Source: CAD feature listing. Evaluate the final solid. Frame: model axes, mm. Give positions to 0.01 mm unless a question says otherwise; leave off trailing zeros. Order: outer loops, then holes, each group sorted by start corner. A loop starts at its lowest first (then second) coordinate and runs counter-clockwise, first axis right, second up.
from build123d import *

# Parameters (mm, degrees)
ESQUISSE1_W             = 40
ESQUISSE1_H             = 17
BOSS_EXTRU_1_DEPTH      = 1
ENL_V_MAT_EXTRU_1_REACH = 45.474
ESQUISSE2_R             = 2.5
BOSS_EXTRU_2_DEPTH      = 8


with BuildPart() as part:
    # Esquisse1 → Boss.-Extru.1 (new body)
    with BuildSketch(Plane.XY):
        with Locations((20, 8.5)):
            Rectangle(ESQUISSE1_W, ESQUISSE1_H)
    extrude(amount=BOSS_EXTRU_1_DEPTH)

    # Esquisse2 → Enlèv. mat.-Extru.1 (cut, up to next)
    with BuildSketch(Plane.XY.offset(1), mode=Mode.PRIVATE) as enl_v_mat_extru_1_sk1:
        with Locations((6.5, 10.5)):
            Circle(ESQUISSE2_R)
    enl_v_mat_extru_1_tool1 = extrude(enl_v_mat_extru_1_sk1.sketch, amount=-ENL_V_MAT_EXTRU_1_REACH, mode=Mode.PRIVATE) & part.part
    # Esquisse2 → Enlèv. mat.-Extru.1 (cut, up to next)
    with BuildSketch(Plane.XY.offset(1), mode=Mode.PRIVATE) as enl_v_mat_extru_1_sk2:
        with Locations((33.5, 10.5)):
            Circle(ESQUISSE2_R)
    enl_v_mat_extru_1_tool2 = extrude(enl_v_mat_extru_1_sk2.sketch, amount=-ENL_V_MAT_EXTRU_1_REACH, mode=Mode.PRIVATE) & part.part
    add(enl_v_mat_extru_1_tool1.solids().sort_by_distance((6.5, 10.5, 1))[0], mode=Mode.SUBTRACT)
    add(enl_v_mat_extru_1_tool2.solids().sort_by_distance((33.5, 10.5, 1))[0], mode=Mode.SUBTRACT)

    # Esquisse3 → Boss.-Extru.2 (add)
    with BuildSketch(Plane.ZY.offset(-8)):
        with BuildLine():
            Line((0, 0), (0, -2))
            ThreePointArc((0, -2), (3.414213562, -3.414213562), (2, 0))
            Line((2, 0), (2, -1))
            ThreePointArc((2, -1), (2.707106781, -2.707106781), (1, -2))
            Line((1, -2), (1, 0))
            Line((1, 0), (0, 0))
        make_face()
    boss_extru_2 = extrude(amount=BOSS_EXTRU_2_DEPTH)

    # Symétrie1: Boss.-Extru.2 across plane
    add(boss_extru_2.mirror(Plane.ZY.offset(-20)))


solid = part.part
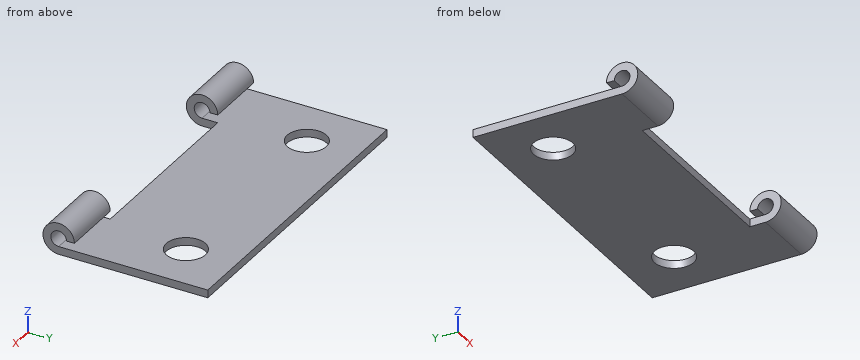
1) Ray query, L1, parallel to Z at x = 35.25, y = -2; L2, parallel to X at y = -1.25, z = 3.35; L3, parallel to Z at x = 37.5, y = 0.75. Return the intervals inside material, ascending.
Checks:
L1: z = 0 to 1, 3 to 4
L2: x = 0 to 8, 32 to 40
L3: z = 0 to 1
2) Section query C-C on z = 3.4. Output: boundary loops of the cut face in (x, y), and give its area (3 significant figures).
Checks:
outline: (0, -3.43) - (8, -3.43) - (8, -0.57) - (0, -0.57) - close; (32, -3.43) - (40, -3.43) - (40, -0.57) - (32, -0.57) - close
area: 45.7 mm2
3) Section query A-A on x = 5. Output: boundary loops of the cut face in (y, z).
Checks:
outline: (-2, 0) - (8.5, 0) - (8.5, 1) - (-2, 1) arc R1 cw (long way) to (-1, 2) - (0, 2) arc R2 ccw (long way) to start; (12.5, 0) - (17, 0) - (17, 1) - (12.5, 1) - close
4) First-contact query: pin 1 Ø2 at (y, z) = (15, 3) entering from +X; pin 2 Ø6 at (x, y) = (12, -1) entering from -Z; pin 3 Ø0.8 at (x, z) = (15.5, 0.5) entering from -Y. Flat tips, straight axial feed; report the tip coordinate or a pass-through.
Checks:
pin 1: passes through
pin 2: stops at z = 0
pin 3: stops at y = 0
5) Section query B-B on y = -2.5. Output: boundary loops of the cut face in (x, z).
Checks:
outline: (0, 0.06) - (8, 0.06) - (8, 1.13) - (0, 1.13) - close; (0, 2.87) - (8, 2.87) - (8, 3.94) - (0, 3.94) - close; (32, 0.06) - (40, 0.06) - (40, 1.13) - (32, 1.13) - close; (32, 2.87) - (40, 2.87) - (40, 3.94) - (32, 3.94) - close
6) Section query D-D on y = 9.5. Output: boundary loops of the cut face in (x, z).
Checks:
outline: (0, 0) - (4.21, 0) - (4.21, 1) - (0, 1) - close; (8.79, 0) - (31.21, 0) - (31.21, 1) - (8.79, 1) - close; (35.79, 0) - (40, 0) - (40, 1) - (35.79, 1) - close
